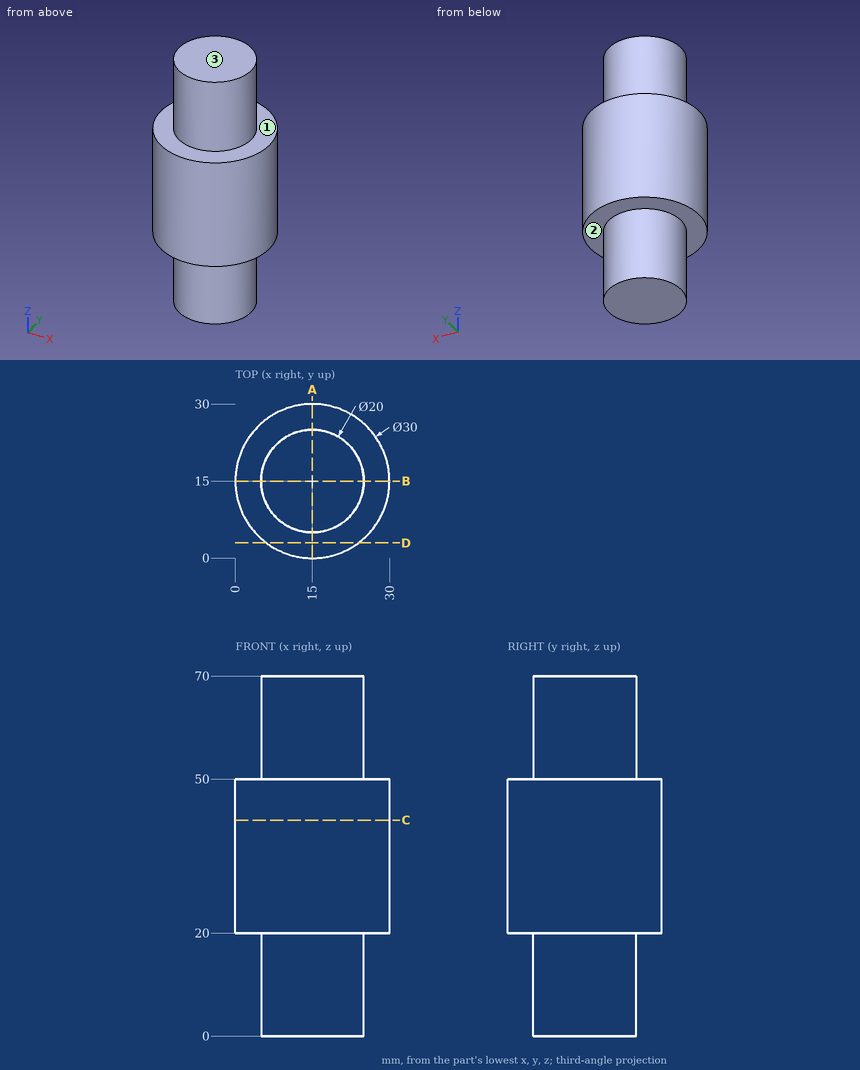
Could you check a few things on this drawing? It's one solid part, dimensions in mm from its lowest x, y, z. A direction names the side the tool comes from. Give positions to 0.01 mm unless a question says otherwise; leave off trailing zeros. Order: outer loops, then holes, each group sorted by start corner. A loop starts at its lowest first (then second) coordinate and runs counter-clockwise, first axis right, second up. Notation, with made-up numbers: (22.25, 45) -> (66.25, 45) arc R19 ccw to (66.25, 73) -> close; hole circle Ø8 at (89.5, 0.5). An arc over 180 degrees is marked (long way). Use CSV: the item, a comma, the result in double quotes. Start each with the question number.
Item 1: I'm going to push flat-ended pins straight in: P1, Ø3, axis at y = 26.5, z = 19, coming from the +X side; P2, Ø6, axis at y = 14.5, z = 60.5, coming from the +X side; P3, Ø5, axis at x = 26.5, z = 32.5, coming from the +Y side. Where does each tip first touch, or does it pass through?
Item 2: Suppose I cut it at A-A (x = 15). List the corners of the cut face in (y, z) for me.
Item 3: Suppose I cut it at C-C (z = 42). List the corners of the cut face in (x, y) for me.
Item 4: If I drill on probe 1 along X at (y, z) = (15.5, 4.5); probe 2 along Z at (x, y) = (9.5, 3.5); probe 3 along Y at (x, z) = (20, 33), over which ranges is the centre line in solid material (lowest first)? Write a range as [from, to].
Item 5: Suppose I cut it at D-D (y = 3). List the corners of the cut face in (x, z) for me.
Item 6: On a 3-axis mill with a long thin cutter (end or side, diameter ignored), from which of +Z, -Z, +X, -X, +Y, -Y can I reach the whole of each face in a straight line? I mean the marked faces 1, 2 and 3. Say none if no direction works.
Answer block:
1,P1,"stops at x = 25.83"
1,P2,"stops at x = 25"
1,P3,"stops at y = 27"
2,outline,"(0, 20) -> (5, 20) -> (5, 0) -> (25, 0) -> (25, 20) -> (30, 20) -> (30, 50) -> (25, 50) -> (25, 70) -> (5, 70) -> (5, 50) -> (0, 50) -> close"
3,outline,"circle Ø30 at (15, 15)"
4,probe 1,"x = [5.01, 24.99]"
4,probe 2,"z = [20, 50]"
4,probe 3,"y = [0.86, 29.14]"
5,outline,"(6, 20) -> (24, 20) -> (24, 50) -> (6, 50) -> close"
6,face 1,"+Z"
6,face 2,"-Z"
6,face 3,"+Z, +X, -X, +Y, -Y"
